Could you check a few things on this drawing? It's one solid part, dimensions in mm from its lowest x, y, z. A direction names the side the tool comes from. Give positions to 0.01 mm unless a question says otherwise; leave off trailing zeros. Write each loop counter-clockwise with the first axis right and the second up, starting at its lowest first coordinate (ties: lowest second). Pieces come first, ordered by that corner, then holes. Notation, with made-up numbers: (3, -23.75) - (38, -23.75) arc R11 ccw to (38, -8.75) - close; hole circle Ø9 at (40.25, 77.5). An arc over 180 degrees is marked (long way). One line per item, written item: value. Start each with the question number.
1) I'm going to push flat-ended pins straight in: P1, Ø3, axis at x = 34.5, z = 6.5, coming from the +Y side; P2, Ø6.5, axis at x = 18, z = 16, coming from the +Y side; P3, Ø8, axis at y = 24.5, z = 11.5, coming from the -X side. Where does each tip first touch, or does it pass through?
2) On a 3-axis mill with a long thin cutter (end or side, diameter ignored), from which of +Z, -Z, +X, -X, +Y, -Y can I reach the whole of each face in a straight line? I mean the marked faces 1, 2, 3 and 4. Say none if no direction works.
3) Imagine slicing it at D-D on x = 20. Write out the boundary of the cut face in (y, z), plus the area to 3 significant figures.
4) Imagine slicing it at A-A on y = 52. Write out the boundary of the cut face in (x, z), plus the area to 3 significant figures.
5) Imagine slicing it at C-C on z = 4.75. Write out the boundary of the cut face in (x, y).
6) Please list where these lines run through material, in increasing order: L1, parallel to Y at x = 17, z = 15.5; L2, parallel to Z at x = 29.5, y = 52; L3, parallel to Y at x = 15.5, z = 8.5. Write a range as [from, to].
7) Imagine slicing it at B-B on x = 5. Write out the boundary of the cut face in (y, z), plus the area to 3 significant figures.
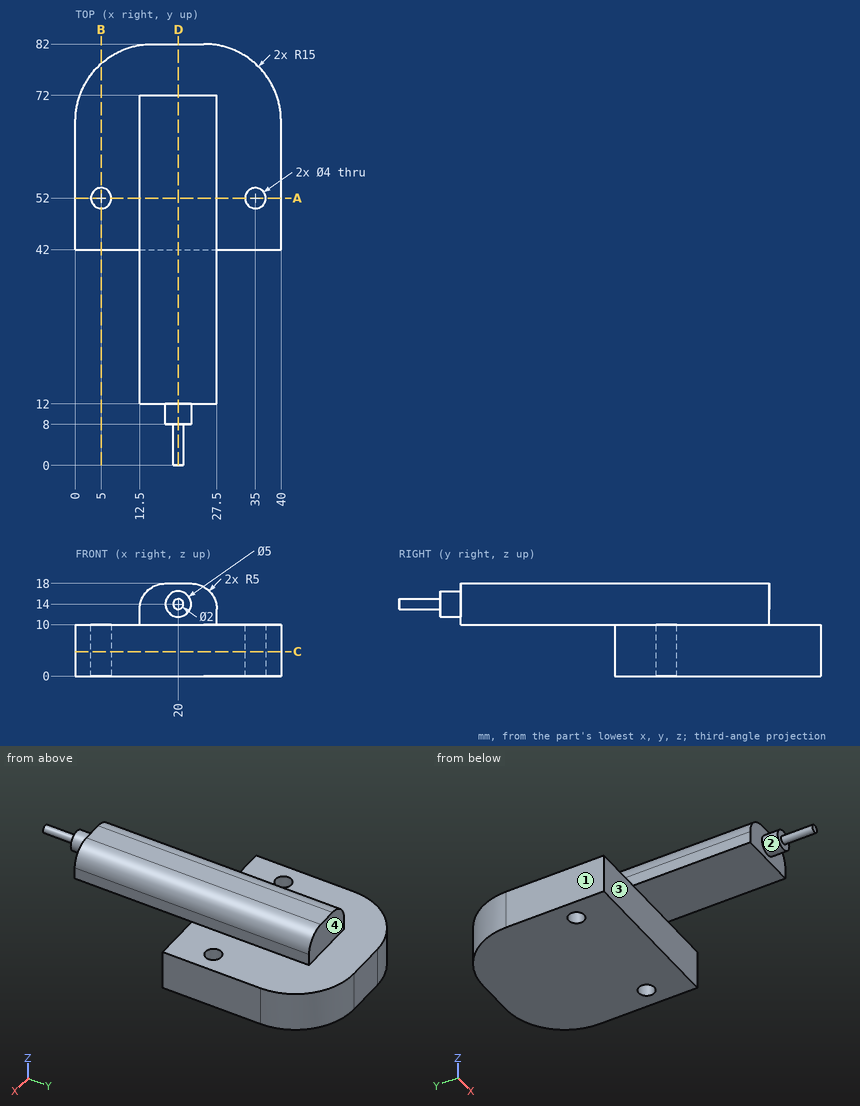
Numbers:
1. P1: y = 79.69
1. P2: y = 72
1. P3: x = 12.5
2. face 1: +Z, -Z, -X, +Y, -Y
2. face 2: -Y
2. face 3: -Z, +X, -X, -Y
2. face 4: +Z, +X, -X, +Y
3. outline: (0, 13) - (8, 13) - (8, 11.5) - (12, 11.5) - (12, 10) - (42, 10) - (42, 0) - (82, 0) - (82, 10) - (72, 10) - (72, 18) - (12, 18) - (12, 16.5) - (8, 16.5) - (8, 15) - (0, 15) - close
3. area: 916 mm^2
4. outline: (0, 0) - (3, 0) - (3, 10) - (0, 10) - close; (7, 0) - (33, 0) - (33, 10) - (27.5, 10) - (27.5, 13) arc R5 ccw to (22.5, 18) - (17.5, 18) arc R5 ccw to (12.5, 13) - (12.5, 10) - (7, 10) - close; (37, 0) - (40, 0) - (40, 10) - (37, 10) - close
4. area: 429 mm^2
5. outline: (0, 42) - (40, 42) - (40, 67) arc R15 ccw to (25, 82) - (15, 82) arc R15 ccw to (0, 67) - close; hole circle Ø4 at (5, 52); hole circle Ø4 at (35, 52)
6. L1: [12, 72]
6. L2: [0, 10]
6. L3: [42, 82]
7. outline: (42, 0) - (50, 0) - (50, 10) - (42, 10) - close; (54, 0) - (78.18, 0) - (78.18, 10) - (54, 10) - close
7. area: 322 mm^2
